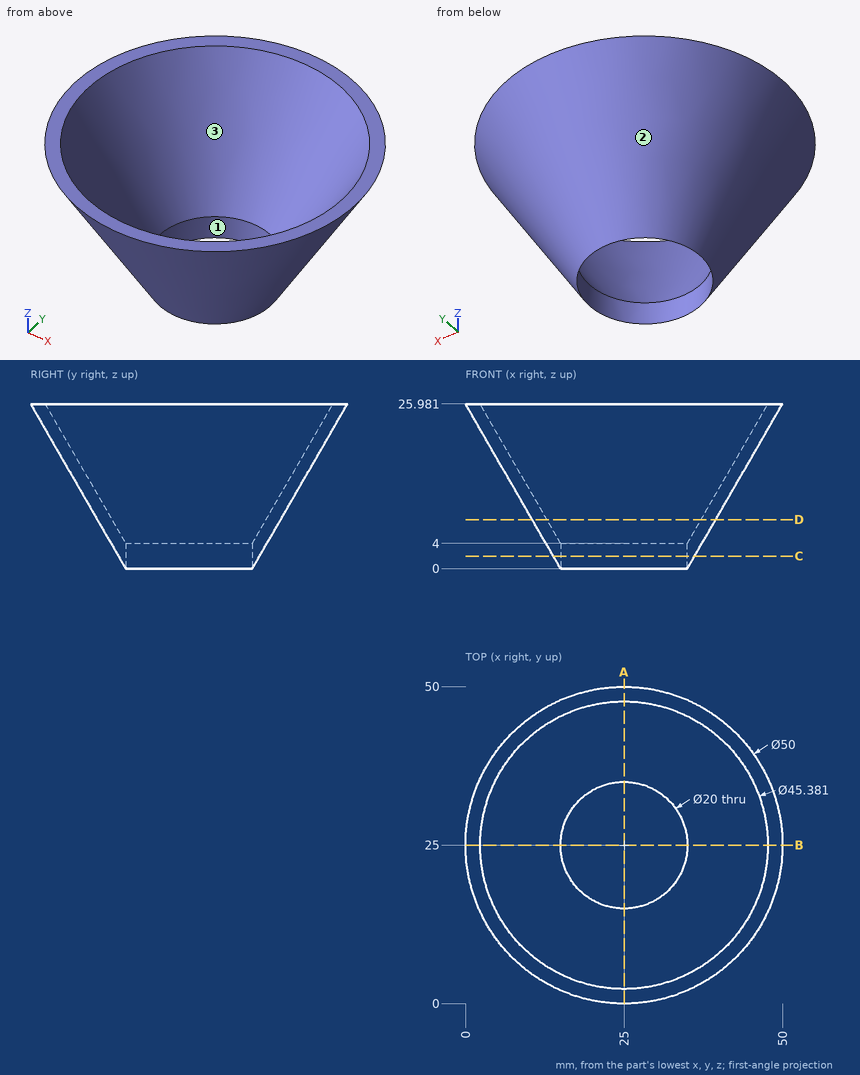
Verification items for this drawing (mm, ordinates from the low corner). Give positions to 0.01 mm unless a question says otherwise; leave off trailing zeros. Write each loop counter-clockwise with the first axis right and the second up, starting at its lowest first coordinate (ties: lowest second). Pieces come first, ordered by that corner, then holes. Notation, with made-up numbers: (5, -33.5) -> (24, -33.5) arc R16 ccw to (24, -22.5) -> close; hole circle Ø11 at (85, 76). An arc over 180 degrees is marked (long way). Write item = value, one per line.
Item 1: Sectioned sample at C-C on z = 2. Record the boundary of the cut face in (x, y) (1 decimal).
Output:
outline = circle Ø22.3 at (25, 25); hole circle Ø20 at (25, 25)
Item 2: Gauge pin test, flat ends, axial feed: pin 1 (10 mm diameter, centred on y = 19.5, z = 18.5, fed in from +X); pin 2 (10 mm diameter, centred on x = 11.5, y = 12.5, fed in from -Z) (1 decimal); pin 3 (8 mm diameter, centred on y = 40, z = 3.5, fed in from +X). Record the tip position at first contact, or that the pin passes through.
Output:
pin_1 = 48.09
pin_2 = 5.9
pin_3 = 31.38
Item 3: Release check for a two-part mould opening along X. For the marked faces 1, 2 and 3 record: +X half, -X half, draft (parallel to the pull), parting line (faces both ways), or undercut.
Output:
face_1 = undercut
face_2 = parting line
face_3 = undercut
Item 4: Sectioned sample at A-A on x = 25. Record the boundary of the cut face in (y, z), and give its area (3 significant figures).
Output:
outline = (0, 25.98) -> (15, 0) -> (15, 4) -> (2.31, 25.98) -> close; (35, 0) -> (50, 25.98) -> (47.69, 25.98) -> (35, 4) -> close
area = 111 mm^2
Item 5: Scan lines: probe 1 along Y at (x, z) = (14.5, 9.5); probe 2 along X at (y, z) = (18, 20.5); probe 3 along X at (y, z) = (25, 1.1) (1 decimal). Record each from-to range of solid material in increasing order. Write a range as from..to.
Output:
probe_1 = 13.62..17.04, 32.96..36.38
probe_2 = 4.32..6.77, 43.23..45.68
probe_3 = 14.4..15, 35..35.6
Item 6: Sectioned sample at D-D on z = 7.75. Record the boundary of the cut face in (x, y) (1 decimal), and give its area (3 significant figures).
Output:
outline = circle Ø28.9 at (25, 25); hole circle Ø24.3 at (25, 25)
area = 193 mm^2
